Geometry: final body of the model. Coordinates: model frame, mm. A direction names the side the tool comes from. Give positions to 0.01 mm unless a question says otherwise; leave off trailing zeros. Loops run counter-clockwise (first coordinate to the right, second up) from the corner with the lowest first, then second, coordinate; pieces in that order, holes last. Notation, with made-up numbers: (-4, -19) - (48, -19) arc R10 cw to (48, -14) - close; hole circle Ø8 at (-21, -35). An arc over 180 degrees is marked (long way). Use one line per item in the form item = value.
```python
from build123d import *

# Parameters (mm, degrees)
SKIZZE1_W                          = 65
SKIZZE1_H                          = 50
AUFSATZ_LINEAR_AUSTRAGEN1_DEPTH    = 3
SKIZZE2_W                          = 65
SKIZZE2_H                          = 50
SKIZZE2_W_2                        = 59
SKIZZE2_H_2                        = 44
AUFSATZ_LINEAR_AUSTRAGEN2_DEPTH    = 23
SKIZZE4_R                          = 2
SKIZZE4_R_2                        = 1
AUFSATZ_LINEAR_AUSTRAGEN3_DEPTH    = 3.5
SCHNITT_LINEAR_AUSTRAGEN1_REACH    = 52
SKIZZE5_R                          = 6.25
VERRUNDUNG1_R                      = 3
F_1_0_1_DURCHMESSER_BOHRUNG1_D     = 1
F_1_0_1_DURCHMESSER_BOHRUNG1_DEPTH = 15
F_1_0_1_DURCHMESSER_BOHRUNG1_TIP   = 0.30043031


with BuildPart() as part:
    # Skizze1 → Aufsatz-Linear austragen1 (new body)
    with BuildSketch(Plane.XY):
        with Locations((32.5, -25)):
            Rectangle(SKIZZE1_W, SKIZZE1_H)
    extrude(amount=AUFSATZ_LINEAR_AUSTRAGEN1_DEPTH)

    # Skizze2 → Aufsatz-Linear austragen2 (add)
    with BuildSketch(Plane.XY.offset(3)):
        with Locations((32.5, -25)):
            Rectangle(SKIZZE2_W, SKIZZE2_H)
        with Locations((32.5, -25)):
            Rectangle(SKIZZE2_W_2, SKIZZE2_H_2, mode=Mode.SUBTRACT)
    extrude(amount=AUFSATZ_LINEAR_AUSTRAGEN2_DEPTH)

    # Skizze4 → Aufsatz-Linear austragen3 (add)
    with BuildSketch(Plane.XY.offset(3)):
        with Locations((7.797786215, -7)):
            Circle(SKIZZE4_R)
        with Locations((7.797786215, -7)):
            Circle(SKIZZE4_R_2, mode=Mode.SUBTRACT)
        with Locations((56.797786215, -7)):
            Circle(SKIZZE4_R)
        with Locations((56.797786215, -7)):
            Circle(SKIZZE4_R_2, mode=Mode.SUBTRACT)
        with Locations((56.797786215, -43)):
            Circle(SKIZZE4_R)
        with Locations((56.797786215, -43)):
            Circle(SKIZZE4_R_2, mode=Mode.SUBTRACT)
        with Locations((7.797786215, -43)):
            Circle(SKIZZE4_R)
        with Locations((7.797786215, -43)):
            Circle(SKIZZE4_R_2, mode=Mode.SUBTRACT)
    extrude(amount=AUFSATZ_LINEAR_AUSTRAGEN3_DEPTH)

    # Skizze5 → Schnitt-Linear austragen1 (cut, up to next)
    with BuildSketch(Plane(origin=(0, 0, 0), x_dir=(1, 0, 0), z_dir=(0, 1, 0)), mode=Mode.PRIVATE) as schnitt_linear_austragen1_sk1:
        with Locations((32.5, -15)):
            Circle(SKIZZE5_R)
    schnitt_linear_austragen1_tool1 = extrude(schnitt_linear_austragen1_sk1.sketch, amount=-SCHNITT_LINEAR_AUSTRAGEN1_REACH, mode=Mode.PRIVATE) & part.part
    add(schnitt_linear_austragen1_tool1.solids().sort_by_distance((32.5, 0, 15))[0], mode=Mode.SUBTRACT)

    # Verrundung1
    verrundung1_edges = [part.edges().sort_by_distance(p)[0] for p in [
        (0, 0, 13),
        (65, 0, 13),
        (65, -50, 13),
        (0, -50, 13),
    ]]
    fillet(verrundung1_edges, radius=VERRUNDUNG1_R)

    # Ø1.0 (1) Durchmesser Bohrung1
    with Locations(Plane.XY.offset(26)):
        with Locations((63, -48), (63, -2), (2, -2), (2, -48)):
            Hole(F_1_0_1_DURCHMESSER_BOHRUNG1_D / 2, depth=F_1_0_1_DURCHMESSER_BOHRUNG1_DEPTH)
            with Locations((0, 0, -(F_1_0_1_DURCHMESSER_BOHRUNG1_DEPTH + F_1_0_1_DURCHMESSER_BOHRUNG1_TIP / 2))):  # 118° drill point
                Cone(0, F_1_0_1_DURCHMESSER_BOHRUNG1_D / 2, F_1_0_1_DURCHMESSER_BOHRUNG1_TIP, mode=Mode.SUBTRACT)


solid = part.part
```
(1) Cut plane C-C (z = 22.5). Return the cut outline in (x, y), plus the area to 3 significant figures.
Solution:
outline = (0, -47) arc R3 ccw to (3, -50) - (62, -50) arc R3 ccw to (65, -47) - (65, -3) arc R3 ccw to (62, 0) - (3, 0) arc R3 ccw to (0, -3) - close; hole circle Ø1 at (2, -48); hole circle Ø1 at (2, -2); hole (3, -47) - (62, -47) - (62, -3) - (3, -3) - close; hole circle Ø1 at (63, -48); hole circle Ø1 at (63, -2)
area = 643 mm2
(2) Pull-direction query (X, two-part tool) for faces 4 (the face through (32, -25, 3)), 5 (the face through (65, -25, 13)), 6 (the face through (32, 0, 7)), 7 (the face through (58.705, -6.399, 4.726)); classes: released by +X, released by -X, zero draft, split by the parting line, or undercut.
Solution:
face_4 = undercut
face_5 = released by +X
face_6 = zero draft
face_7 = undercut
(3) Access query for faces 1 (the face through (0.86, -0.9, 12.82)), 2 (the face through (27.54, -1.48, 18.8)), 3 (the face through (57, -7, 3)). Directions: +Z, -Z, +X, -X, +Y, -Y. A direction counts if a zero-diameter tool reaches every point of the face in a straight line with its end or side. Return the directions, or none.
Solution:
face_1 = +Z, -Z, -X, +Y
face_2 = +Y
face_3 = +Z
(4) Pin query (flat end, axial travel): P1, Ø1.2, axis at x = 7.5, y = -7.5, coming from the +Z side; P2, Ø2, axis at x = 48, y = -10, coming from the +Z side. Return the tip coordinate at first contact, or that it passes through.
Solution:
P1 = 6.5
P2 = 3
(5) Cut plane D-D (x = 41). Return the cut outline in (y, z), plus the area to 3 significant figures.
Solution:
outline = (-50, 0) - (0, 0) - (0, 26) - (-3, 26) - (-3, 3) - (-47, 3) - (-47, 26) - (-50, 26) - close
area = 288 mm2
(6) Cut plane A-A (x = 32.5). Return the cut outline in (y, z).
Solution:
outline = (-50, 0) - (0, 0) - (0, 8.75) - (-3, 8.75) - (-3, 3) - (-47, 3) - (-47, 26) - (-50, 26) - close; (-3, 21.25) - (0, 21.25) - (0, 26) - (-3, 26) - close
(7) Material intervals for L1, parallel to X at y = -31.5, z = 4.5; L2, parallel to Y at x = 52, z = 6.75; L3, parallel to Y at x = 63, z = 18, sorted ascending. Write a range as from..to.
Solution:
L1 = 0..3, 62..65
L2 = -50..-47, -3..0
L3 = -49.83..-48.5, -47.5..-2.5, -1.5..-0.17
(8) Cut plane B-B (y = -43). Return the cut outline in (x, z).
Solution:
outline = (0, 0) - (65, 0) - (65, 26) - (62, 26) - (62, 3) - (58.8, 3) - (58.8, 6.5) - (57.8, 6.5) - (57.8, 3) - (55.8, 3) - (55.8, 6.5) - (54.8, 6.5) - (54.8, 3) - (9.8, 3) - (9.8, 6.5) - (8.8, 6.5) - (8.8, 3) - (6.8, 3) - (6.8, 6.5) - (5.8, 6.5) - (5.8, 3) - (3, 3) - (3, 26) - (0, 26) - close
